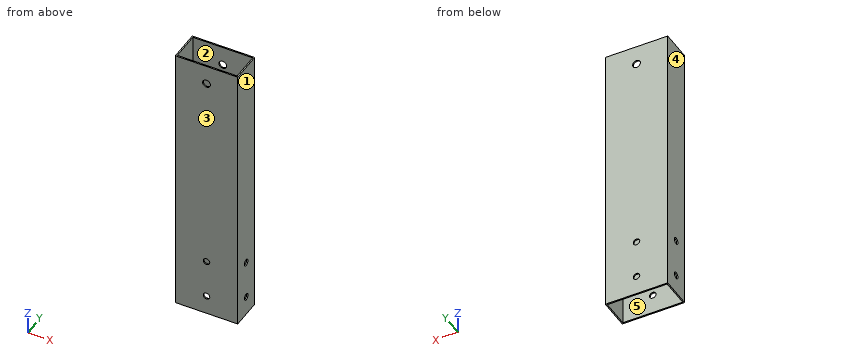
```python
from build123d import *

# Parameters (mm, degrees)
SKETCH2_W           = 48
SKETCH2_H           = 24
SKETCH2_W_2         = 46
SKETCH2_H_2         = 22
BOSS_EXTRUDE1_DEPTH = 240
SKETCH4_R           = 3
CUT_EXTRUDE1_DEPTH  = 240
CUT_EXTRUDE3_DEPTH  = 240
CUT_EXTRUDE4_DEPTH  = 240
SKETCH8_W           = 48
SKETCH8_H           = 25
CUT_EXTRUDE5_DEPTH  = 25


with BuildPart() as part:
    # Sketch2 → Boss-Extrude1 (new body)
    with BuildSketch(Plane.XY):
        Rectangle(SKETCH2_W, SKETCH2_H)
        Rectangle(SKETCH2_W_2, SKETCH2_H_2, mode=Mode.SUBTRACT)
    extrude(amount=BOSS_EXTRUDE1_DEPTH)

    # Sketch4 → Cut-Extrude1 (cut)
    with BuildSketch(Plane.XZ.offset(12)):
        with Locations((0, 200)):
            Circle(SKETCH4_R)
    extrude(amount=-CUT_EXTRUDE1_DEPTH, mode=Mode.SUBTRACT)

    # Sketch5 → Cut-Extrude3 (cut)
    with BuildSketch(Plane.XZ.offset(12)):
        with BuildLine():
            ThreePointArc((2.5, 45), (1.767766953, 46.767766953), (0, 47.5))
            Line((0, 47.5), (0, 42.5))
            ThreePointArc((0, 42.5), (1.767766953, 43.232233047), (2.5, 45))
        make_face()
        with BuildLine():
            Line((0, 42.5), (0, 47.5))
            ThreePointArc((0, 47.5), (-2.5, 45), (0, 42.5))
        make_face()
        with BuildLine():
            ThreePointArc((0, 17.5), (-2.5, 15), (0, 12.5))
            Line((0, 12.5), (0, 17.5))
        make_face()
        with BuildLine():
            Line((0, 17.5), (0, 12.5))
            ThreePointArc((0, 12.5), (1.767766953, 13.232233047), (2.5, 15))
            ThreePointArc((2.5, 15), (1.767766953, 16.767766953), (0, 17.5))
        make_face()
    extrude(amount=-CUT_EXTRUDE3_DEPTH, mode=Mode.SUBTRACT)

    # Sketch7 → Cut-Extrude4 (cut)
    with BuildSketch(Plane(origin=(24, 0, 0), x_dir=(0, 0, -1), z_dir=(1, 0, 0))):
        with BuildLine():
            ThreePointArc((-42.5, 0), (-45, 2.5), (-47.5, 0))
            Line((-47.5, 0), (-42.5, 0))
        make_face()
        with BuildLine():
            Line((-42.5, 0), (-47.5, 0))
            ThreePointArc((-47.5, 0), (-45, -2.5), (-42.5, 0))
        make_face()
        with BuildLine():
            ThreePointArc((-17.5, 0), (-15, -2.5), (-12.5, 0))
            Line((-12.5, 0), (-17.5, 0))
        make_face()
        with BuildLine():
            Line((-17.5, 0), (-12.5, 0))
            ThreePointArc((-12.5, 0), (-15, 2.5), (-17.5, 0))
        make_face()
    extrude(amount=-CUT_EXTRUDE4_DEPTH, mode=Mode.SUBTRACT)

    # Sketch8 → Cut-Extrude5 (cut, through all)
    with BuildSketch(Plane.XZ.offset(12)):
        with Locations((0, 227.5)):
            Rectangle(SKETCH8_W, SKETCH8_H)
    extrude(amount=-CUT_EXTRUDE5_DEPTH, mode=Mode.SUBTRACT)


solid = part.part
```
Check sheet for the modelled part. Datum: model origin and axes. Units: mm. Face numbers are marked on the shaded views. A direction names the side the tool comes from. Round coordinates to 2 decimals unless told otherwise and drop trailing zeros. Order: outer loops, then holes, each group sorted by start corner. A loop starts at its lowest first (then second) coordinate and runs counter-clockwise, first axis right, second up. Notation, with made-up numbers: (30, -30.5) - (42, -30.5) arc R31 ccw to (42, 8.5) - close; hole circle Ø1 at (72.5, -10). An arc over 180 degrees is marked (long way). Answer as CSV lines item,"result". Start each with the question number.
1) Draft check along X on the marked faces 1, 2 and 3. Enter one of: +X half, -X half, draft (parallel to the pull), parting line (faces both ways), or undercut.
2) Depth check by flat-ended pin: pin 1 (4.5 mm diameter, centred on y = 0, z = 15, fed in from +X). Enter the tip coordinate at first touch or a pass-through.
3) Section check A-A (z = 200). Record the cut outline in (x, y).
4) Tool access check on the marked faces 4 and 5. Record the directions out of +Z, -Z, +X, -X, +Y, -Y that give a thin tool (end or side, any length) a straight path to the whole face; none if there is none.
5) Section check C-C (x = 5). Record the cut outline in (y, z), then the cut area to 3 significant figures.
6) Section check B-B (y = -5.5). Record the cut outline in (x, z).
7) Section check D-D (z = 35.5). Record the cut outline in (x, y).
8) Scan lines: probe 1 along Z at (x, y) = (0, -11.6); probe 2 along Y at (x, z) = (-23.65, 15); probe 3 along Y at (x, z) = (17, 21). Record each from-to range of solid material in increasing order.
Determined:
1,face 1,"+X half"
1,face 2,"undercut"
1,face 3,"draft"
2,pin 1,"through"
3,outline,"(-24, -12) - (-3, -12) - (-3, -11) - (-23, -11) - (-23, 11) - (-3, 11) - (-3, 12) - (-24, 12) - close; (3, -12) - (24, -12) - (24, 12) - (3, 12) - (3, 11) - (23, 11) - (23, -11) - (3, -11) - close"
4,face 4,"+Z, -Z, -X, +Y, -Y"
4,face 5,"+Z, -Z"
5,outline,"(-12, 0) - (-11, 0) - (-11, 215) - (-12, 215) - close; (11, 0) - (12, 0) - (12, 215) - (11, 215) - close"
5,area,"430 mm^2"
6,outline,"(-24, 0) - (-23, 0) - (-23, 215) - (-24, 215) - close; (23, 0) - (24, 0) - (24, 215) - (23, 215) - close"
7,outline,"(-24, -12) - (24, -12) - (24, 12) - (-24, 12) - close; hole (-23, -11) - (23, -11) - (23, 11) - (-23, 11) - close"
8,probe 1,"0 to 12.5, 17.5 to 42.5, 47.5 to 197, 203 to 215"
8,probe 2,"-12 to -2.5, 2.5 to 12"
8,probe 3,"-12 to -11, 11 to 12"
